from build123d import *

# Parameters (mm, degrees)
SKETCH1_R           = 2.5
BOSS_EXTRUDE1_DEPTH = 7
CUT_EXTRUDE1_DEPTH  = 3.5
SKETCH7_R           = 6
SKETCH7_R_2         = 2.5
BOSS_EXTRUDE2_DEPTH = 5.25
SKETCH8_R           = 6
SKETCH8_R_2         = 2.5
BOSS_EXTRUDE3_DEPTH = 1.75


with BuildPart() as part:
    # Sketch1 → Boss-Extrude1 (new body)
    with BuildSketch(Plane(origin=(0, 0, 0), x_dir=(0, 0, -1), z_dir=(1, 0, 0))):
        with BuildLine():
            Line((28.813942393, -15.5), (-28.813942393, -15.5))
            ThreePointArc((-28.813942393, -15.5), (-31.041774365, -14.76649875), (-32.398076983, -12.852941176))
            ThreePointArc((-32.398076983, -12.852941176), (-34.636038969, -9.136038969), (-38.352941176, -6.898076983))
            ThreePointArc((-38.352941176, -6.898076983), (-40.26649875, -5.541774365), (-41, -3.313942393))
            Line((-41, -3.313942393), (-41, 3.313942393))
            ThreePointArc((-41, 3.313942393), (-40.26649875, 5.541774365), (-38.352941176, 6.898076983))
            ThreePointArc((-38.352941176, 6.898076983), (-34.636038969, 9.136038969), (-32.398076983, 12.852941176))
            ThreePointArc((-32.398076983, 12.852941176), (-31.041774365, 14.76649875), (-28.813942393, 15.5))
            Line((-28.813942393, 15.5), (28.813942393, 15.5))
            ThreePointArc((28.813942393, 15.5), (31.041774365, 14.76649875), (32.398076983, 12.852941176))
            ThreePointArc((32.398076983, 12.852941176), (34.636038969, 9.136038969), (38.352941176, 6.898076983))
            ThreePointArc((38.352941176, 6.898076983), (40.26649875, 5.541774365), (41, 3.313942393))
            Line((41, 3.313942393), (41, -3.313942393))
            ThreePointArc((41, -3.313942393), (40.26649875, -5.541774365), (38.352941176, -6.898076983))
            ThreePointArc((38.352941176, -6.898076983), (34.636038969, -9.136038969), (32.398076983, -12.852941176))
            ThreePointArc((32.398076983, -12.852941176), (31.041774365, -14.76649875), (28.813942393, -15.5))
        make_face()
        with Locations((-32, 0)):
            Circle(SKETCH1_R, mode=Mode.SUBTRACT)
        with Locations((32, 0)):
            Circle(SKETCH1_R, mode=Mode.SUBTRACT)
    extrude(amount=BOSS_EXTRUDE1_DEPTH)

    # Sketch6 → Cut-Extrude1 (cut)
    with BuildSketch(Plane(origin=(7, 0, 0), x_dir=(0, 0, -1), z_dir=(1, 0, 0))):
        with BuildLine():
            Line((28.813942393, 12), (-28.813942393, 12))
            ThreePointArc((-28.813942393, 12), (-28.962464524, 11.951099917), (-29.052884699, 11.823529412))
            ThreePointArc((-29.052884699, 11.823529412), (-32.161165235, 6.661165235), (-37.323529412, 3.552884699))
            ThreePointArc((-37.323529412, 3.552884699), (-37.451099917, 3.462464524), (-37.5, 3.313942393))
            Line((-37.5, 3.313942393), (-37.5, -3.313942393))
            ThreePointArc((-37.5, -3.313942393), (-37.451099917, -3.462464524), (-37.323529412, -3.552884699))
            ThreePointArc((-37.323529412, -3.552884699), (-32.161165235, -6.661165235), (-29.052884699, -11.823529412))
            ThreePointArc((-29.052884699, -11.823529412), (-28.962464524, -11.951099917), (-28.813942393, -12))
            Line((-28.813942393, -12), (28.813942393, -12))
            ThreePointArc((28.813942393, -12), (28.962464524, -11.951099917), (29.052884699, -11.823529412))
            ThreePointArc((29.052884699, -11.823529412), (32.161165235, -6.661165235), (37.323529412, -3.552884699))
            ThreePointArc((37.323529412, -3.552884699), (37.451099917, -3.462464524), (37.5, -3.313942393))
            Line((37.5, -3.313942393), (37.5, 3.313942393))
            ThreePointArc((37.5, 3.313942393), (37.451099917, 3.462464524), (37.323529412, 3.552884699))
            ThreePointArc((37.323529412, 3.552884699), (32.161165235, 6.661165235), (29.052884699, 11.823529412))
            ThreePointArc((29.052884699, 11.823529412), (28.962464524, 11.951099917), (28.813942393, 12))
        make_face()
    extrude(amount=-CUT_EXTRUDE1_DEPTH, mode=Mode.SUBTRACT)

    # Sketch7 → Boss-Extrude2 (add)
    with BuildSketch(Plane(origin=(3.5, 0, 0), x_dir=(0, 0, -1), z_dir=(1, 0, 0))):
        with Locations((32, 0)):
            Circle(SKETCH7_R)
        with Locations((32, 0)):
            Circle(SKETCH7_R_2, mode=Mode.SUBTRACT)
    boss_extrude2 = extrude(amount=-BOSS_EXTRUDE2_DEPTH)

    # Mirror1: Boss-Extrude2 across plane
    add(boss_extrude2.mirror(Plane.XY))

    # Sketch8 → Boss-Extrude3 (add)
    with BuildSketch(Plane(origin=(3.5, 0, 0), x_dir=(0, 0, -1), z_dir=(1, 0, 0))):
        with Locations((32, 0)):
            Circle(SKETCH8_R)
        with Locations((32, 0)):
            Circle(SKETCH8_R_2, mode=Mode.SUBTRACT)
    boss_extrude3 = extrude(amount=BOSS_EXTRUDE3_DEPTH)

    # Mirror2: Boss-Extrude3 across plane
    add(boss_extrude3.mirror(Plane.XY))


solid = part.part
Part model, mm, in its own coordinate system. A direction names the side the tool comes from. Give positions to 0.01 mm unless a question says otherwise; leave off trailing zeros. Write each loop counter-clockwise with the first axis right and the second up, starting at its lowest first coordinate (ties: lowest second). Pieces come first, ordered by that corner, then holes.
1) Cut at C-C on z = -17. Write the cut outline in (x, y).
Resolved:
outline: (0, -15.5) - (7, -15.5) - (7, -12) - (3.5, -12) - (3.5, 12) - (7, 12) - (7, 15.5) - (0, 15.5) - close
2) Cut at D-D on y = -8. Write the cut outline in (x, z), then the cut area to 3 significant figures.
Resolved:
outline: (0, -36.03) - (7, -36.03) - (7, -31) - (3.5, -31) - (3.5, 31) - (7, 31) - (7, 36.03) - (0, 36.03) - close
area: 287 mm2
3) Probe L1, parallel to Z at x = 2.4, y = 0; L2, parallel to Y at x = -0.5, z = 32; L3, parallel to Y at x = 6.5, z = 11. List the from-to ranges inside material, lowest first.
Resolved:
L1: z = -41 to -34.5, -29.5 to 29.5, 34.5 to 41
L2: y = -6 to -2.5, 2.5 to 6
L3: y = -15.5 to -12, 12 to 15.5
4) Cut at A-A on x = 1.75. Write the cut outline in (y, z).
Resolved:
outline: (-15.5, -28.81) arc R3.75 ccw to (-12.85, -32.4) arc R9 cw to (-6.9, -38.35) arc R3.75 ccw to (-3.31, -41) - (3.31, -41) arc R3.75 ccw to (6.9, -38.35) arc R9 cw to (12.85, -32.4) arc R3.75 ccw to (15.5, -28.81) - (15.5, 28.81) arc R3.75 ccw to (12.85, 32.4) arc R9 cw to (6.9, 38.35) arc R3.75 ccw to (3.31, 41) - (-3.31, 41) arc R3.75 ccw to (-6.9, 38.35) arc R9 cw to (-12.85, 32.4) arc R3.75 ccw to (-15.5, 28.81) - close; hole circle Ø5 at (0, -32); hole circle Ø5 at (0, 32)
5) Pin check, flat tips, straight feed: pin 1 (6 mm diameter, centred on y = 2.5, z = 15.5, fed in from +X); pin 2 (6.5 mm diameter, centred on y = 0, z = -32, fed in from +X); pin 3 (3 mm diameter, centred on y = 9, z = 30.5, fed in from -X). Stop position of each tip, or through.
Resolved:
pin 1: stops at x = 3.5
pin 2: stops at x = 5.25
pin 3: stops at x = 0
6) Which spindle directions (+Z, -Z, +X, -X, +Y, -Y) get a long thin tool onto all of the face, cutting with end or side? Do faces 1 (the face through (0, 0, -1)), 2 (the face through (-1.75, 0, -35)), 3 (the face through (5, 12, 0)). Say none if no direction does.
Resolved:
face 1: -X
face 2: +Z, -Z, -X, +Y, -Y
face 3: +X
7) Two-plate mould, pull along Z, no slides. Class faces 4 (the face through (4, 0, -26)), 5 (the face through (3.45, -9.18, 34.59)), 6 (the face through (6, 0, -37.5)), 7 (the face through (3.45, -9.09, -34.68)): released by +Z, released by -Z, zero draft, split by the parting line, or undercut.
Resolved:
face 4: undercut
face 5: released by +Z
face 6: undercut
face 7: released by -Z
